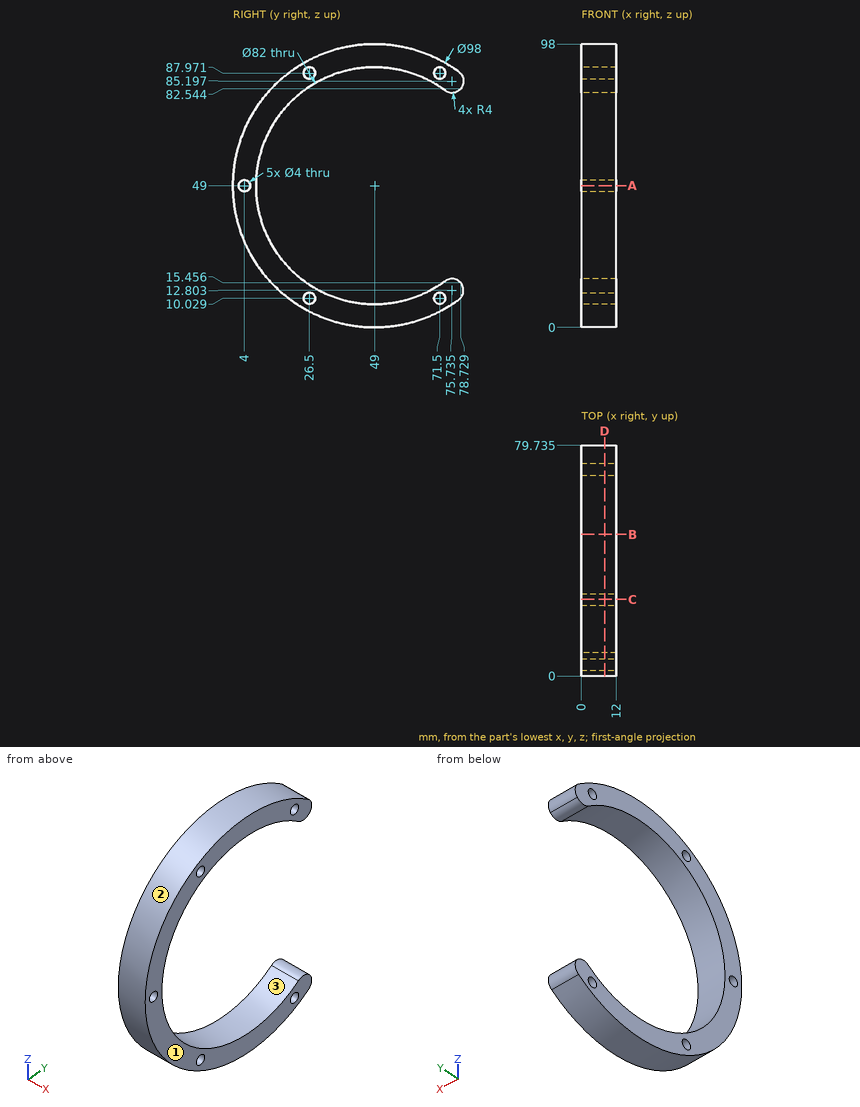
Geometry: see drawing. Coordinates: mm, zero at the bounding-box minimum. Coordinates: 2 decimals unless noted, no trailing zeros. Write each loop counter-clockwise with the first axis right and the second up, starting at its lowest first coordinate (ties: lowest second). Pieces come first, ordered by that corner, then holes. Notation, with made-up numbers: M 62,-17.75 L 66,-17.75 A19 ccw 66,13.25 Z; hole C 54.25,21.25 d8. An arc over 180 degrees is marked long. Use CSV: the item, a comma, the result in double quotes. Start each with the question number.
1. Cut plane C-C on y = 26.5. Return the cut outline in (x, z) (1 decimal), plus the area to 3 significant figures.
2. Cut plane A-A on z = 49. Return the cut outline in (x, y).
3. Cut plane B-B on y = 49. Return the cut outline in (x, z).
4. Ray query, probe 1 along Z at (x, y) = (7, 66) (1 decimal); probe 2 along Z at (x, y) = (7.25, 38.5); probe 3 along Y at (x, z) = (11, 13.5) (1 decimal). Return the intervals inside material, ascending.
5. Mould query, pull axis Y, two halves, no side actions, for the marked faces 1, 2 and 3. Classes: pulls with the +Y half, pulls with the -Y half, needs draft (parallel to the pull), parting line crosses it, or undercut.
6. Cut plane D-D on x = 8. Count the separate pieces of the cut face and the enclosed holes in it, plus the area to 3 significant figures.
7. First-contact query: P1, Ø1.5, axis at x = 8, y = 57.5, coming from the +Z side; P2, Ø1, axis at x = 3, y = 17.5, coming from the -Z side; P3, Ø3, axis at y = 71.5, z = 87.97, coming from the +X side; P4, Ø6, axis at x = 4.5, z = 62, coming from the +Y side. Flat tips, straight axial feed; report the tip coordinate or a pass-through.
Entries:
1,outline,"M 0,5.5 L 12,5.5 L 12,8 L 0,8 Z; M 0,12 L 12,12 L 12,14.7 L 0,14.7 Z; M 0,83.3 L 12,83.3 L 12,86 L 0,86 Z; M 0,90 L 12,90 L 12,92.5 L 0,92.5 Z"
1,area,"126 mm²"
2,outline,"M 0,0 L 12,0 L 12,2 L 0,2 Z; M 0,6 L 12,6 L 12,8 L 0,8 Z"
3,outline,"M 0,0 L 12,0 L 12,8 L 0,8 Z; M 0,90 L 12,90 L 12,98 L 0,98 Z"
4,probe 1,"3 to 11.7, 86.3 to 95"
4,probe 2,"1.14 to 9.37, 88.63 to 96.86"
4,probe 3,"15.2 to 28.5, 69.5 to 79.7"
5,face 1,"needs draft"
5,face 2,"parting line crosses it"
5,face 3,"undercut"
6,separate pieces,"1"
6,enclosed holes,"5"
6,area,"1,580 mm²"
7,P1,"z = 97.38"
7,P2,"z = 11.05"
7,P3,"through"
7,P4,"y = 11.25"
